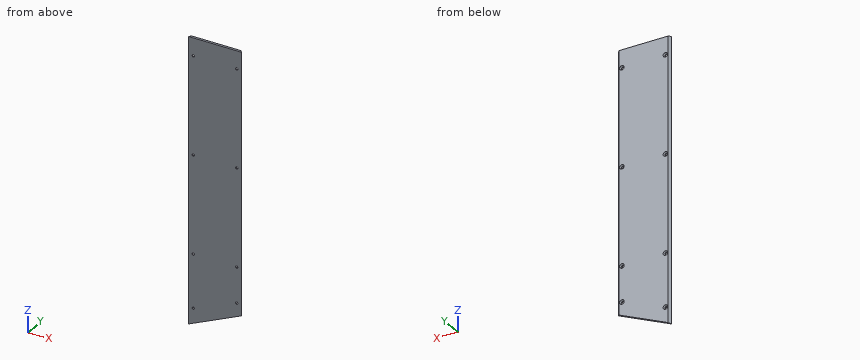
```python
from build123d import *

# Parameters (mm, degrees)
SKETCH1_W                                     = 152.4
SKETCH1_H                                     = 1219.2
BOSS_EXTRUDE1_DEPTH                           = 6.35
CSK_FOR_1_4_FLAT_HEAD_MACHINE_SCREW1_AT_COUNT = 2
CSK_FOR_1_4_FLAT_HEAD_MACHINE_SCREW1_AT_PITCH = 123.825
CSK_FOR_1_4_FLAT_HEAD_MACHINE_SCREW1_2_COUNT  = 2
CSK_FOR_1_4_FLAT_HEAD_MACHINE_SCREW1_2_PITCH  = 305.609212271
CSK_FOR_1_4_FLAT_HEAD_MACHINE_SCREW1_3_COUNT  = 2
CSK_FOR_1_4_FLAT_HEAD_MACHINE_SCREW1_3_PITCH  = 572.354846773
CSK_FOR_1_4_FLAT_HEAD_MACHINE_SCREW1_4_COUNT  = 2
CSK_FOR_1_4_FLAT_HEAD_MACHINE_SCREW1_4_PITCH  = 847.296801968
CSK_FOR_1_4_FLAT_HEAD_MACHINE_SCREW1_5_COUNT  = 2
CSK_FOR_1_4_FLAT_HEAD_MACHINE_SCREW1_5_PITCH  = 1124.438700252
CSK_FOR_1_4_FLAT_HEAD_MACHINE_SCREW1_6_COUNT  = 2
CSK_FOR_1_4_FLAT_HEAD_MACHINE_SCREW1_6_PITCH  = 279.4
CSK_FOR_1_4_FLAT_HEAD_MACHINE_SCREW1_7_COUNT  = 2
CSK_FOR_1_4_FLAT_HEAD_MACHINE_SCREW1_7_PITCH  = 558.8
CSK_FOR_1_4_FLAT_HEAD_MACHINE_SCREW1_8_COUNT  = 2
CSK_FOR_1_4_FLAT_HEAD_MACHINE_SCREW1_8_PITCH  = 838.2
CSK_FOR_1_4_FLAT_HEAD_MACHINE_SCREW1_9_COUNT  = 2
CSK_FOR_1_4_FLAT_HEAD_MACHINE_SCREW1_9_PITCH  = 1117.6
CHAMFER1_SIZE                                 = 6.35
CUT_EXTRUDE1_DEPTH                            = 1229.704489493
CSK_FOR_1_4_FLAT_HEAD_MACHINE_SCREW2_AT_COUNT = 2
CSK_FOR_1_4_FLAT_HEAD_MACHINE_SCREW2_AT_PITCH = 133.840467068


with BuildPart() as part:
    # Sketch1 → Boss-Extrude1 (new body)
    with BuildSketch(Plane(origin=(0, 0, 0), x_dir=(1, 0, 0), z_dir=(0, 1, 0))):
        with Locations((76.2, 609.6)):
            Rectangle(SKETCH1_W, SKETCH1_H)
    extrude(amount=BOSS_EXTRUDE1_DEPTH)

    # Sketch3 → CSK for 1/4 Flat Head Machine Screw1 (revolve, cut)
    with BuildSketch(Plane(origin=(14.2875, 6.35, -1168.4), x_dir=(0, 0, 1), z_dir=(1, 0, 0))):
        Polygon((0, 0), (0, 6.35), (3.3782, 6.35), (3.3782, 3.520932584), (6.4389, 0), align=None)
    csk_for_1_4_flat_head_machine_screw1 = revolve(axis=Axis((14.2875, 12.7, -1168.4), (0, -1, 0)), mode=Mode.SUBTRACT)

    # CSK for 1/4 Flat Head Machine Screw1 at: CSK for 1/4 Flat Head Machine Screw1 ×2
    with Locations(*[(i * CSK_FOR_1_4_FLAT_HEAD_MACHINE_SCREW1_AT_PITCH, 0, 0) for i in range(1, CSK_FOR_1_4_FLAT_HEAD_MACHINE_SCREW1_AT_COUNT)]):
        add(csk_for_1_4_flat_head_machine_screw1, mode=Mode.SUBTRACT)

    # CSK for 1_4 Flat Head Machine Screw1 2: CSK for 1/4 Flat Head Machine Screw1 ×2
    with Locations(*[Vector(0.405174304399354, 0, 0.9142394560805718) * (i * CSK_FOR_1_4_FLAT_HEAD_MACHINE_SCREW1_2_PITCH) for i in range(1, CSK_FOR_1_4_FLAT_HEAD_MACHINE_SCREW1_2_COUNT)]):
        add(csk_for_1_4_flat_head_machine_screw1, mode=Mode.SUBTRACT)

    # CSK for 1_4 Flat Head Machine Screw1 3: CSK for 1/4 Flat Head Machine Screw1 ×2
    with Locations(*[Vector(0.21634306182267615, 0, 0.9763174071997232) * (i * CSK_FOR_1_4_FLAT_HEAD_MACHINE_SCREW1_3_PITCH) for i in range(1, CSK_FOR_1_4_FLAT_HEAD_MACHINE_SCREW1_3_COUNT)]):
        add(csk_for_1_4_flat_head_machine_screw1, mode=Mode.SUBTRACT)

    # CSK for 1_4 Flat Head Machine Screw1 4: CSK for 1/4 Flat Head Machine Screw1 ×2
    with Locations(*[Vector(0.1461412337594335, 0, 0.9892637362176331) * (i * CSK_FOR_1_4_FLAT_HEAD_MACHINE_SCREW1_4_PITCH) for i in range(1, CSK_FOR_1_4_FLAT_HEAD_MACHINE_SCREW1_4_COUNT)]):
        add(csk_for_1_4_flat_head_machine_screw1, mode=Mode.SUBTRACT)

    # CSK for 1_4 Flat Head Machine Screw1 5: CSK for 1/4 Flat Head Machine Screw1 ×2
    with Locations(*[Vector(0.11012160998392527, 0, 0.9939181208804618) * (i * CSK_FOR_1_4_FLAT_HEAD_MACHINE_SCREW1_5_PITCH) for i in range(1, CSK_FOR_1_4_FLAT_HEAD_MACHINE_SCREW1_5_COUNT)]):
        add(csk_for_1_4_flat_head_machine_screw1, mode=Mode.SUBTRACT)

    # CSK for 1_4 Flat Head Machine Screw1 6: CSK for 1/4 Flat Head Machine Screw1 ×2
    with Locations(*[(0, 0, i * CSK_FOR_1_4_FLAT_HEAD_MACHINE_SCREW1_6_PITCH) for i in range(1, CSK_FOR_1_4_FLAT_HEAD_MACHINE_SCREW1_6_COUNT)]):
        add(csk_for_1_4_flat_head_machine_screw1, mode=Mode.SUBTRACT)

    # CSK for 1_4 Flat Head Machine Screw1 7: CSK for 1/4 Flat Head Machine Screw1 ×2
    with Locations(*[(0, 0, i * CSK_FOR_1_4_FLAT_HEAD_MACHINE_SCREW1_7_PITCH) for i in range(1, CSK_FOR_1_4_FLAT_HEAD_MACHINE_SCREW1_7_COUNT)]):
        add(csk_for_1_4_flat_head_machine_screw1, mode=Mode.SUBTRACT)

    # CSK for 1_4 Flat Head Machine Screw1 8: CSK for 1/4 Flat Head Machine Screw1 ×2
    with Locations(*[(0, 0, i * CSK_FOR_1_4_FLAT_HEAD_MACHINE_SCREW1_8_PITCH) for i in range(1, CSK_FOR_1_4_FLAT_HEAD_MACHINE_SCREW1_8_COUNT)]):
        add(csk_for_1_4_flat_head_machine_screw1, mode=Mode.SUBTRACT)

    # CSK for 1_4 Flat Head Machine Screw1 9: CSK for 1/4 Flat Head Machine Screw1 ×2
    with Locations(*[(0, 0, i * CSK_FOR_1_4_FLAT_HEAD_MACHINE_SCREW1_9_PITCH) for i in range(1, CSK_FOR_1_4_FLAT_HEAD_MACHINE_SCREW1_9_COUNT)]):
        add(csk_for_1_4_flat_head_machine_screw1, mode=Mode.SUBTRACT)

    # Chamfer1
    chamfer1_edges = [part.edges().sort_by_distance(p)[0] for p in [
        (0, 6.35, -609.6),
        (152.4, 6.35, -609.6),
    ]]
    chamfer(chamfer1_edges, length=CHAMFER1_SIZE - 0.0001)  # a hair under: the kernel refuses the full size

    # Sketch4 → Cut-Extrude1 (cut, through all)
    with BuildSketch(Plane(origin=(0, 6.35, 0), x_dir=(1, 0, 0), z_dir=(0, 1, 0))):
        Polygon((152.4, 742.95), (0, 810.802851641), (0, 1219.2), (152.4, 1219.2), align=None)
    extrude(amount=-CUT_EXTRUDE1_DEPTH, mode=Mode.SUBTRACT)

    # Sketch6 → CSK for 1/4 Flat Head Machine Screw2 (revolve, cut)
    with BuildSketch(Plane(origin=(14.2875, 6.35, -762), x_dir=(0, 0, 1), z_dir=(1, 0, 0))):
        Polygon((0, 0), (0, 6.35), (3.3782, 6.35), (3.3782, 3.520932584), (6.4389, 0), align=None)
    csk_for_1_4_flat_head_machine_screw2 = revolve(axis=Axis((14.2875, 12.7, -762), (0, -1, 0)), mode=Mode.SUBTRACT)

    # CSK for 1/4 Flat Head Machine Screw2 at: CSK for 1/4 Flat Head Machine Screw2 ×2
    with Locations(*[Vector(0.9251686183747461, 0, 0.3795563562563057) * (i * CSK_FOR_1_4_FLAT_HEAD_MACHINE_SCREW2_AT_PITCH) for i in range(1, CSK_FOR_1_4_FLAT_HEAD_MACHINE_SCREW2_AT_COUNT)]):
        add(csk_for_1_4_flat_head_machine_screw2, mode=Mode.SUBTRACT)


solid = part.part
```
Geometry: final body of the model. Coordinates: model frame, mm. Coordinates: 2 decimals unless noted, no trailing zeros. Order: outer loops, then holes, each group sorted by start corner. A loop starts at its lowest first (then second) coordinate and runs counter-clockwise, first axis right, second up. Notation, with made-up numbers: (-37.75, -6) -> (-18.75, -6) arc R22 cw to (-18.75, 27) -> close; hole circle Ø3 at (73.25, 78). An arc over 180 degrees is marked (long way). Write item = value, one per line.
(1) Pin query (flat end, axial travel): pin 1 Ø2 at (y, z) = (4, -561) entering from +X; pin 2 Ø11 at (x, z) = (14.29, -50.8) entering from -Y; pin 3 Ø8 at (x, z) = (14.29, -330.2) entering from +Y; pin 4 Ø3 at (x, y) = (96, 3.5) entering from -Z. Return the tip coordinate at first contact, or that it passes through.
Solved:
pin_1 = 149.4
pin_2 = 0
pin_3 = 3.55
pin_4 = -768.73
(2) Cut plane C-C on x = 79.5. Return loops of the section in (y, z), plus the area to 3 significant figures.
Solved:
outline = (0, -775.41) -> (6.35, -775.41) -> (6.35, 0) -> (0, 0) -> close
area = 4,920 mm²
(3) Cut plane B-B on y = 1.5. Count the separate pieces of the cut face and the enclosed holes in it, plus the area to 3 significant figures.
Solved:
separate_pieces = 1
enclosed_holes = 8
area = 116,000 mm²
(4) Line query: line 1 (X direction, y = 1.1, z = -330.2); line 2 (X direction, y = 6.25, z = -328); line 3 (Z direction, x = 15, y = 1). Output: solid intervals per line, ascending.
Solved:
line_1 = 1.1 to 10.91, 17.67 to 134.73, 141.49 to 151.3
line_2 = 6.25 to 8.33, 20.25 to 132.15, 144.07 to 146.15
line_3 = -804.12 to -765.3, -758.7 to -612.9, -606.3 to -333.5, -326.9 to -54.1, -47.5 to 0
